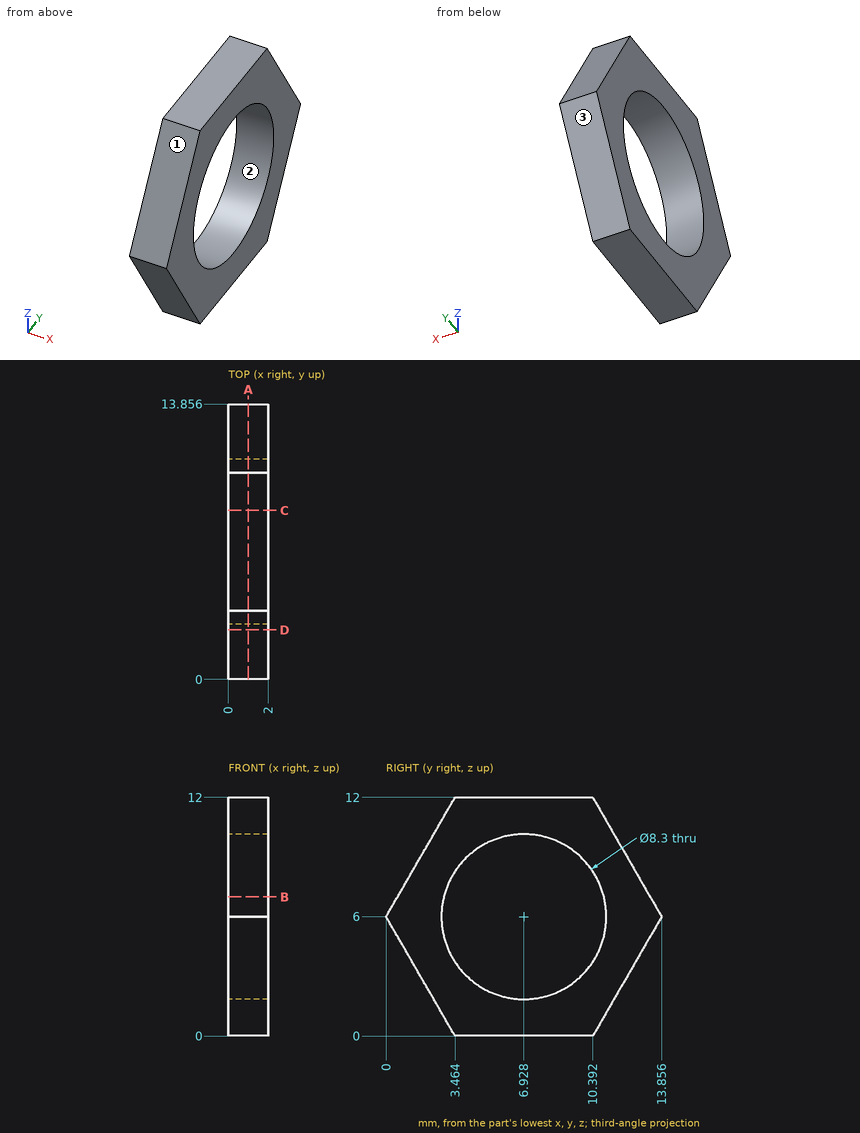
Geometry check sheet. Reference: drawing and pictorial views, mm from the part's lowest x, y, z. Coordinates: 2 decimals unless noted, no trailing zeros. Order: outer loops, then holes, each group sorted by start corner. A loop starts at its lowest first (then second) coordinate and runs counter-clockwise, first axis right, second up. Notation, with made-up numbers: (31.5, 73) - (82.5, 73) arc R12 ccw to (82.5, 89) - close; hole circle Ø6 at (3.5, 52). An arc over 180 degrees is marked (long way). One line per item, written item: value.
(1) Sectioned sample at A-A (x = 1). Enter the section's corners in (y, z).
Data:
outline: (0, 6) - (3.46, 0) - (10.39, 0) - (13.86, 6) - (10.39, 12) - (3.46, 12) - close; hole circle Ø8.3 at (6.93, 6)
(2) Thickness scan on probe 1 along Y at (x, z) = (0.25, 6.5); probe 2 along Y at (x, z) = (1.4, 2.5) (1 decimal); probe 3 along Z at (x, y) = (1.7, 10). Record the ranges inside material, lowest first. Write a range as from..to.
Data:
probe 1: y = 0.29..2.81, 11.05..13.57
probe 2: y = 2..4.7, 9.2..11.8
probe 3: z = 0..3.21, 8.79..12
(3) Sectioned sample at D-D (y = 2.5). Enter the section's corners in (x, z), and give its area (3 significant figures).
Data:
outline: (0, 1.67) - (2, 1.67) - (2, 10.33) - (0, 10.33) - close
area: 17.3 mm^2
(4) Sectioned sample at C-C (y = 8.5). Enter the section's corners in (x, z).
Data:
outline: (0, 0) - (2, 0) - (2, 2.16) - (0, 2.16) - close; (0, 9.84) - (2, 9.84) - (2, 12) - (0, 12) - close
(5) Depth check by flat-ended pin: pin 1 Ø1 at (y, z) = (7.5, 3.5) entering from +X; pin 2 Ø5 at (y, z) = (10.5, 8) entering from -X. Enter the tip coordinate at first touch or a pass-through.
Data:
pin 1: passes through
pin 2: stops at x = 0
(6) Release check for a two-part mould opening along Y. For the marked faces 1, 2 and 3 record: +Y half, -Y half, draft (parallel to the pull), parting line (faces both ways), or undercut.
Data:
face 1: -Y half
face 2: undercut
face 3: +Y half
(7) Sectioned sample at B-B (z = 7). Enter the section's corners in (x, y).
Data:
outline: (0, 0.58) - (2, 0.58) - (2, 2.9) - (0, 2.9) - close; (0, 10.96) - (2, 10.96) - (2, 13.28) - (0, 13.28) - close
